Geometry check sheet. Reference: the model listing, model coordinates, mm. A direction names the side the tool comes from. Give positions to 0.01 mm unless a question says otherwise; leave off trailing zeros. Loops run counter-clockwise (first coordinate to the right, second up) from the corner with the lowest first, then second, coordinate; pieces in that order, holes last. Notation, with made-up numbers: (4.25, -24.75) -> (15.25, -24.75) arc R21 ccw to (15.25, 1.25) -> close; hole circle Ø10 at (4.25, 76). An arc over 180 degrees is marked (long way). Answer as a JSON object with one key per item and string values.
from build123d import *

# Parameters (mm, degrees)
F1_DEPTH = 82


with BuildPart() as f1:
    # F0 (on Top) → F1 (new body)
    with BuildSketch(Plane.XY):
        with BuildLine():
            Line((10.5, 19.5), (-10.5, 19.5))
            ThreePointArc((-10.5, 19.5), (-11.56066, 19.06066), (-12, 18))
            Line((-12, 18), (-12, -18))
            ThreePointArc((-12, -18), (-11.56066, -19.06066), (-10.5, -19.5))
            Line((-10.5, -19.5), (-7.5, -19.5))
            Line((-7.5, -19.5), (-7.5, -21.5))
            ThreePointArc((-7.5, -21.5), (-7.207107, -22.207107), (-6.5, -22.5))
            Line((-6.5, -22.5), (6.5, -22.5))
            ThreePointArc((6.5, -22.5), (7.207107, -22.207107), (7.5, -21.5))
            Line((7.5, -21.5), (7.5, -19.5))
            Line((7.5, -19.5), (10.5, -19.5))
            ThreePointArc((10.5, -19.5), (11.56066, -19.06066), (12, -18))
            Line((12, -18), (12, 18))
            ThreePointArc((12, 18), (11.56066, 19.06066), (10.5, 19.5))
        make_face()
    extrude(amount=F1_DEPTH)


solid = f1.part
1) Section check A-A on z = 66.5. Record the cut outline in (x, y), plus the area to 3 significant figures.
Geometry check:
{"outline": "(-12, -18) arc R1.5 ccw to (-10.5, -19.5) -> (-7.5, -19.5) -> (-7.5, -21.5) arc R1 ccw to (-6.5, -22.5) -> (6.5, -22.5) arc R1 ccw to (7.5, -21.5) -> (7.5, -19.5) -> (10.5, -19.5) arc R1.5 ccw to (12, -18) -> (12, 18) arc R1.5 ccw to (10.5, 19.5) -> (-10.5, 19.5) arc R1.5 ccw to (-12, 18) -> close", "area": "979 mm2"}
2) Material ranges on line 1 along Y through (x, z) = (10.5, 35); line 2 along Y through (x, z) = (6.75, 14.5), recorded low to high. Write a range as from..to.
Geometry check:
{"line 1": "y = -19.5..19.5", "line 2": "y = -22.47..19.5"}
3) Depth check by flat-ended pin: P1, Ø2, axis at x = 8, y = 7, coming from the -Z side; P2, Ø3.5, axis at x = -8.5, z = 51.5, coming from the -Y side; P3, Ø2, axis at y = -20, z = 36.5, coming from the +X side; P4, Ø1, axis at y = -20.5, z = 28.5, coming from the -X side. Enter the tip coordinate at first touch or a pass-through.
Geometry check:
{"P1": "stops at z = 0", "P2": "stops at y = -22.47", "P3": "stops at x = 11.62", "P4": "stops at x = -7.5"}
4) Section check B-B on x = -8.5. Record the cut outline in (y, z), plus the area to 3 significant figures.
Geometry check:
{"outline": "(-19.5, 0) -> (19.5, 0) -> (19.5, 82) -> (-19.5, 82) -> close", "area": "3,200 mm2"}
5) Tool access check on faces 1 (the face through (0, -22.5, 40)), 2 (the face through (-7.5, -20, 40)), 3 (the face through (7.5, -21, 40)). Record the directions out of +Z, -Z, +X, -X, +Y, -Y that give a thin tool (end or side, any length) a straight path to the whole face; none if there is none.
Geometry check:
{"face 1": "+Z, -Z, +X, -X, -Y", "face 2": "+Z, -Z, -X, -Y", "face 3": "+Z, -Z, +X, -Y"}
